from build123d import *

# Parameters (mm, degrees)
F0_W      = 184.4983883202
F0_H      = 97.9466736317
F1_DEPTH  = 50.8
F2_W      = 48.7498342991
F2_H      = 32.1726370603
F3_DEPTH  = 51.816
F5_DEPTH  = 152.4
F6_DEPTH  = 97.79
F8_DEPTH  = 200.914
F9_W      = 64.6597607993
F9_H      = 21.533165127
F10_DEPTH = 2540
F12_DEPTH = 25.4
F13_W     = 34.1657865793
F13_H     = 12.4993889213
F14_DEPTH = 177.8
F15_R     = 8.0143887739
F16_DEPTH = 381
F15_R_2   = 8.6578968481
F17_DEPTH = 381
F15_R_3   = 7.6783249055
F18_DEPTH = 381
F15_R_4   = 7.5555874341
F19_DEPTH = 381


with BuildPart() as f1:
    # F0 (on Top) → F1 (new body)
    with BuildSketch(Plane.XY):
        with Locations((33.5375722498, 25.2984389663)):
            Rectangle(F0_W, F0_H)
    extrude(amount=F1_DEPTH)

    # F2 (on face) → F3 (cut)
    with BuildSketch(Plane.XY.offset(50.8)):
        with Locations((101.4118492603, -7.5885793194)):
            Rectangle(F2_W, F2_H)
    extrude(amount=-F3_DEPTH, mode=Mode.SUBTRACT)

    # F5 (cut): a face of the model
    f5_faces = [f1.faces().sort_by_distance(p)[0] for p in [
        (101.4118492603, 8.4977392107, 25.4),
    ]]
    extrude(f5_faces, amount=-F5_DEPTH, mode=Mode.SUBTRACT)

    # F4 (on face) → F6 (join)
    with BuildSketch(Plane.XZ.offset(23.6748978496)):
        Polygon((126.6083866358, 0), (77.0369321108, 35.8533561641), (77.0369321108, 0), align=None)
    extrude(amount=-F6_DEPTH)

    # F7 (on face) → F8 (cut)
    with BuildSketch(Plane.XZ.offset(23.6748978496)):
        Polygon((56.3714504242, 50.8), (77.0369321108, 35.8533561641), (77.0369321108, 50.8), align=None)
    extrude(amount=-F8_DEPTH, mode=Mode.SUBTRACT)

    # F9 (on face) → F10 (cut)
    with BuildSketch(Plane.XZ.offset(23.6748978496)):
        with Locations((-26.3817415107, 10.7665825635)):
            Rectangle(F9_W, F9_H)
    extrude(amount=-F10_DEPTH, mode=Mode.SUBTRACT)

    # F11 (on face) → F12 (join)
    with BuildSketch(Plane.XZ.offset(23.6748978496)):
        Polygon((5.9481388889, 21.533165127), (5.9481388889, 0), (70.435055404, 0), (70.435055404, 40.6282702591), (56.3714504242, 50.8), (5.9481388889, 50.8), align=None)
    extrude(amount=F12_DEPTH)

    # F13 (on face) → F14 (cut)
    with BuildSketch(Plane(origin=(-58.7116219103, 0, 0), x_dir=(0, -1, 0), z_dir=(-1, 0, 0))):
        with Locations((-27.9484977946, 44.5503055394)):
            Rectangle(F13_W, F13_H)
    extrude(amount=-F14_DEPTH, mode=Mode.SUBTRACT)

    # F15 (on face) → F16 (cut)
    with BuildSketch(Plane(origin=(-58.7116219103, 0, 0), x_dir=(0, -1, 0), z_dir=(-1, 0, 0))):
        with Locations((-57.373650372, 30.5959098041)):
            Circle(F15_R)
    extrude(amount=-F16_DEPTH, mode=Mode.SUBTRACT)

    # F15 (on face) → F17 (cut)
    with BuildSketch(Plane(origin=(-58.7116219103, 0, 0), x_dir=(0, -1, 0), z_dir=(-1, 0, 0))):
        with Locations((3.9370707236, 32.0339165628)):
            Circle(F15_R_2)
    extrude(amount=-F17_DEPTH, mode=Mode.SUBTRACT)

    # F15 (on face) → F18 (cut)
    with BuildSketch(Plane(origin=(-58.7116219103, 0, 0), x_dir=(0, -1, 0), z_dir=(-1, 0, 0))):
        with Locations((3.9370707236, 13.242979534)):
            Circle(F15_R_3)
    extrude(amount=-F18_DEPTH, mode=Mode.SUBTRACT)

    # F15 (on face) → F19 (cut)
    with BuildSketch(Plane(origin=(-58.7116219103, 0, 0), x_dir=(0, -1, 0), z_dir=(-1, 0, 0))):
        with Locations((-57.373650372, 11.7202522233)):
            Circle(F15_R_4)
    extrude(amount=-F19_DEPTH, mode=Mode.SUBTRACT)


solid = f1.part
Build history of the part. All positions in model axes, mm. A direction names the side the tool comes from. Give positions to 0.01 mm unless a question says otherwise; leave off trailing zeros. Write each loop counter-clockwise with the first axis right and the second up, starting at its lowest first coordinate (ties: lowest second). Pieces come first, ordered by that corner, then holes. Notation, with made-up numbers: (-27, -21) - (23, -21) arc R18 cw to (23, 1) - close; hole circle Ø6 at (-27, 67.25). An arc over 180 degrees is marked (long way). Use one line per item in the form item = value. Start each with the question number.
1. Probe line 1 (Y direction, x = 20, z = 24.5); line 2 (Y direction, x = 98, z = 18); line 3 (Y direction, x = -30, z = 48). List the from-to ranges inside material, lowest first. Write a range as [from, to].
2. Band-saw the part on B-B on y = 56. Write the cut outline in (x, z), plus the area to 3 significant figures.
3. Band-saw the part on D-D on x = 10.5. Write the cut outline in (y, z).
4. Band-saw the part on A-A on z = 27.5. Write the cut outline in (x, y).
5. 3-axis set-ups, long thin cutter, end or side, ignore diameter. For faces 1 (the face through (-27, -23.675, 36)), 2 (the face through (-27, 25, 21.533)), 3 (the face through (86, -23.675, 12)), 4 (the face through (7, 28, 38.301)): which of +Z, -Z, +X, -X, +Y, -Y reach the whole face in a straight line?
6. Drop flat-ended pins along their axis: pin 1 Ø12 at (y, z) = (-15.5, 41.5) entering from +X; pin 2 Ø19.5 at (y, z) = (57.37, 11.72) entering from -X; pin 3 Ø1 at (x, z) = (86.5, 7) entering from +Y. Give the stop position or say it passes through.
7. Band-saw the part on C-C on x = -15. Write the cut outline in (y, z), plus the area to 3 significant figures.
8. Two-plate mould, pull along Z, no slides. Class faces 5 (the face through (17.37, 59.11, 22.77)), 6 (the face through (7, 10.866, 44)), 7 (the face through (62.718, 59.012, 4.344)), 8 (the face through (91.982, 27.167, 25.044)): released by +Z, released by -Z, zero draft, split by the parting line, or undercut.
Conclusion:
q1.line_1 = [-49.07, -8.2], [0.33, 52.17], [62.58, 74.27]
q1.line_2 = [-23.67, -9.96], [2.09, 53.17], [61.58, 74.12]
q1.line_3 = [-23.67, 10.87], [45.03, 74.27]
q2.outline = (-58.71, 21.53) - (5.95, 21.53) - (5.95, 19.15) - (100.13, 19.15) - (95.22, 22.7) - (-58.71, 22.7) - close; (-58.71, 38.49) - (73.39, 38.49) - (56.37, 50.8) - (-58.71, 50.8) - close; (5.95, 0) - (126.61, 0) - (120.68, 4.29) - (5.95, 4.29) - close
q2.area = 2,430 mm²
q3.outline = (-49.07, 0) - (74.27, 0) - (74.27, 50.8) - (45.03, 50.8) - (45.03, 38.3) - (10.87, 38.3) - (10.87, 50.8) - (-49.07, 50.8) - close; hole circle Ø17.32 at (-3.94, 32.03); hole circle Ø15.36 at (-3.94, 13.24); hole circle Ø16.03 at (57.37, 30.6); hole circle Ø15.11 at (57.37, 11.72)
q4.outline = (-58.71, -23.67) - (5.95, -23.67) - (5.95, -49.07) - (70.44, -49.07) - (70.44, -23.67) - (88.59, -23.67) - (88.59, -11.31) - (-58.71, -11.31) - close; (-58.71, 3.44) - (88.59, 3.44) - (88.59, 49.98) - (-58.71, 49.98) - close; (-58.71, 64.77) - (88.59, 64.77) - (88.59, 74.12) - (77.04, 74.12) - (77.04, 74.27) - (-58.71, 74.27) - close
q5.face_1 = +Z, -Z, -X, -Y
q5.face_2 = -Z, -X, +Y, -Y
q5.face_3 = +Z, -Z, +X, -Y
q5.face_4 = +Z, +X, -X
q6.pin_1 = 77.53
q6.pin_2 = 5.95
q6.pin_3 = 74.12
q7.outline = (-23.67, 21.53) - (74.27, 21.53) - (74.27, 50.8) - (45.03, 50.8) - (45.03, 38.3) - (10.87, 38.3) - (10.87, 50.8) - (-23.67, 50.8) - close; hole circle Ø17.32 at (-3.94, 32.03); hole circle Ø16.03 at (57.37, 30.6)
q7.area = 2,000 mm²
q8.face_5 = undercut
q8.face_6 = zero draft
q8.face_7 = undercut
q8.face_8 = released by +Z
